```python
from build123d import *

# Parameters (mm, degrees)
CUT_EXTRUDE1_DEPTH      = 13.124355653
CUT_EXTRUDE1_DEPTH_BACK = 13.124355653
SKETCH2_R               = 4.7625
CUT_EXTRUDE2_DEPTH      = 12.14982483
CUT_EXTRUDE2_DEPTH_BACK = 12.14982483
SKETCH3_W               = 0.678207446
SKETCH3_H               = 0.99055699


with BuildPart() as part:
    # Sketch1 → Revolve1 (revolve)
    with BuildSketch(Plane(origin=(0, 0, 0), x_dir=(1, 0, 0), z_dir=(0, 1, 0))):
        with BuildLine():
            Line((0, 7), (0, -7))
            ThreePointArc((0, -7), (-7, 0), (0, 7))
        make_face()
    revolve(axis=Axis((0, 0, -7), (0, 0, 1)))

    # Sketch2 → Cut-Extrude1 (cut, two sides: drawn at the far end of the back side and taken through both)
    with BuildSketch(Plane.XY.offset(-CUT_EXTRUDE1_DEPTH_BACK)):
        Circle(SKETCH2_R)
    extrude(amount=CUT_EXTRUDE1_DEPTH + CUT_EXTRUDE1_DEPTH_BACK, mode=Mode.SUBTRACT)

    # Sketch3 → Cut-Extrude2 (cut, two sides: drawn at the far end of the back side and taken through both)
    with BuildSketch(Plane(origin=(0, 0, 0), x_dir=(0, 0, -1), z_dir=(1, 0, 0)).offset(-CUT_EXTRUDE2_DEPTH_BACK)):
        with Locations((-5.13016508, 0)):
            Rectangle(SKETCH3_W, SKETCH3_H)
    extrude(amount=CUT_EXTRUDE2_DEPTH + CUT_EXTRUDE2_DEPTH_BACK, mode=Mode.SUBTRACT)


solid = part.part
```
The model under review builds one solid part; all positions refer to its coordinate system, in mm. Round coordinates to 2 decimals unless told otherwise and drop trailing zeros. Loops run counter-clockwise (first coordinate to the right, second up) from the corner with the lowest first, then second, coordinate; pieces in that order, holes last. Notation, with made-up numbers: (82.25, 69) -> (135.25, 69) arc R15 cw to (135.25, 91) -> close; hole circle Ø4 at (-34, 36). An arc over 180 degrees is marked (long way). Answer as a JSON object with one key per item and string values. Group by question number.
1) We need section B-B on y = 0. Write out the cut boundary in (x, z).
2) We need section A-A on x = 0. Write out the cut boundary in (y, z), then the cut area to 3 significant figures.
3) We need section C-C on z = 0. Write out the cut boundary in (x, y) (1 decimal), then the cut area to 3 significant figures.
4) For pin 1 Ø4 at (y, z) = (-1, -2) entering from +X; pin 2 Ø6 at (y, z) = (-5.5, -0.5) entering from -X; pin 3 Ø5 at (y, z) = (3.5, 2) entering from -X, all flat-tipped, find the tip position at first contact; note any pin that passes through.
5) We need section D-D on y = 6. Write out the cut boundary in (x, z), then the cut area to 3 significant figures.
6) For line 1 (X direction, y = -0.5, z = 1); line 2 (X direction, y = -1.25, z = -0.5); line 3 (Y direction, x = 0, z = -2.25), list the stretches that pass through material, from the lowest coordinate up. Write a range as [from, to].
Result set:
{
 "1": {"outline": "(-5.1, 4.79) arc R7 ccw to (-4.76, -5.13) -> (-4.76, 4.79) -> close; (4.76, -5.13) arc R7 ccw to (5.1, 4.79) -> (4.76, 4.79) -> close"},
 "2": {"outline": "(-4.76, -5.13) -> (-4.76, 5.13) arc R7 ccw to start; (4.76, -5.13) arc R7 ccw to (4.76, 5.13) -> close", "area": "31.7 mm²"},
 "3": {"outline": "circle Ø14 at (0, 0); hole circle Ø9.5 at (0, 0)", "area": "82.7 mm²"},
 "4": {"pin 1": "x = 7", "pin 2": "x = -6.53", "pin 3": "x = -6.83"},
 "5": {"outline": "circle Ø7.21 at (0, 0)", "area": "40.8 mm²"},
 "6": {"line 1": "[-6.91, -4.74], [4.74, 6.91]", "line 2": "[-6.87, -4.6], [4.6, 6.87]", "line 3": "[-6.63, -4.76], [4.76, 6.63]"}
}
